from build123d import *

# Parameters (mm, degrees)
BOSS_EXTRUDE1_DEPTH = 5
SKETCH2_R           = 1.75
BOSS_EXTRUDE2_DEPTH = 6
CUT_EXTRUDE1_REACH  = 54.111
SKETCH3_R           = 1.75


with BuildPart() as part:
    # Sketch1 → Boss-Extrude1 (new body)
    with BuildSketch(Plane(origin=(0, 0, 0), x_dir=(1, 0, 0), z_dir=(0, 1, 0))):
        with BuildLine():
            Line((0, 0), (50, 0))
            Line((50, 0), (50, 11.2))
            Line((50, 11.2), (49.7, 11.2))
            ThreePointArc((49.7, 11.2), (49.38158785, 11.33158785), (49.25, 11.65))
            ThreePointArc((49.25, 11.65), (49.089793883, 12.579390672), (48.625, 13.4))
            Line((48.625, 13.4), (47.875, 13.4))
            ThreePointArc((47.875, 13.4), (47.410206117, 12.579390672), (47.25, 11.65))
            ThreePointArc((47.25, 11.65), (47.11841215, 11.33158785), (46.8, 11.2))
            Line((46.8, 11.2), (45.8, 11.2))
            ThreePointArc((45.8, 11.2), (45.48158785, 11.33158785), (45.35, 11.65))
            ThreePointArc((45.35, 11.65), (45.189793883, 12.579390672), (44.725, 13.4))
            Line((44.725, 13.4), (43.975, 13.4))
            ThreePointArc((43.975, 13.4), (43.510206117, 12.579390672), (43.35, 11.65))
            ThreePointArc((43.35, 11.65), (43.21841215, 11.33158785), (42.9, 11.2))
            Line((42.9, 11.2), (41.9, 11.2))
            ThreePointArc((41.9, 11.2), (41.58158785, 11.33158785), (41.45, 11.65))
            ThreePointArc((41.45, 11.65), (41.289793883, 12.579390672), (40.825, 13.4))
            Line((40.825, 13.4), (40.075, 13.4))
            ThreePointArc((40.075, 13.4), (39.610206117, 12.579390672), (39.45, 11.65))
            ThreePointArc((39.45, 11.65), (39.31841215, 11.33158785), (39, 11.2))
            Line((39, 11.2), (38, 11.2))
            ThreePointArc((38, 11.2), (37.68158785, 11.33158785), (37.55, 11.65))
            ThreePointArc((37.55, 11.65), (37.389793883, 12.579390672), (36.925, 13.4))
            Line((36.925, 13.4), (36.175, 13.4))
            ThreePointArc((36.175, 13.4), (35.710206117, 12.579390672), (35.55, 11.65))
            ThreePointArc((35.55, 11.65), (35.41841215, 11.33158785), (35.1, 11.2))
            Line((35.1, 11.2), (34.1, 11.2))
            ThreePointArc((34.1, 11.2), (33.78158785, 11.33158785), (33.65, 11.65))
            ThreePointArc((33.65, 11.65), (33.489793883, 12.579390672), (33.025, 13.4))
            Line((33.025, 13.4), (32.275, 13.4))
            ThreePointArc((32.275, 13.4), (31.810206117, 12.579390672), (31.65, 11.65))
            ThreePointArc((31.65, 11.65), (31.51841215, 11.33158785), (31.2, 11.2))
            Line((31.2, 11.2), (30.2, 11.2))
            ThreePointArc((30.2, 11.2), (29.88158785, 11.33158785), (29.75, 11.65))
            ThreePointArc((29.75, 11.65), (29.589793883, 12.579390672), (29.125, 13.4))
            Line((29.125, 13.4), (28.375, 13.4))
            ThreePointArc((28.375, 13.4), (27.910206117, 12.579390672), (27.75, 11.65))
            ThreePointArc((27.75, 11.65), (27.61841215, 11.33158785), (27.3, 11.2))
            Line((27.3, 11.2), (26.3, 11.2))
            ThreePointArc((26.3, 11.2), (25.98158785, 11.33158785), (25.85, 11.65))
            ThreePointArc((25.85, 11.65), (25.689793883, 12.579390672), (25.225, 13.4))
            Line((25.225, 13.4), (24.475, 13.4))
            ThreePointArc((24.475, 13.4), (24.010206117, 12.579390672), (23.85, 11.65))
            ThreePointArc((23.85, 11.65), (23.71841215, 11.33158785), (23.4, 11.2))
            Line((23.4, 11.2), (22.4, 11.2))
            ThreePointArc((22.4, 11.2), (22.08158785, 11.33158785), (21.95, 11.65))
            ThreePointArc((21.95, 11.65), (21.789793883, 12.579390672), (21.325, 13.4))
            Line((21.325, 13.4), (20.575, 13.4))
            ThreePointArc((20.575, 13.4), (20.110206117, 12.579390672), (19.95, 11.65))
            ThreePointArc((19.95, 11.65), (19.81841215, 11.33158785), (19.5, 11.2))
            Line((19.5, 11.2), (18.5, 11.2))
            ThreePointArc((18.5, 11.2), (18.18158785, 11.33158785), (18.05, 11.65))
            ThreePointArc((18.05, 11.65), (17.889793883, 12.579390672), (17.425, 13.4))
            Line((17.425, 13.4), (16.675, 13.4))
            ThreePointArc((16.675, 13.4), (16.210206117, 12.579390672), (16.05, 11.65))
            ThreePointArc((16.05, 11.65), (15.91841215, 11.33158785), (15.6, 11.2))
            Line((15.6, 11.2), (14.6, 11.2))
            ThreePointArc((14.6, 11.2), (14.28158785, 11.33158785), (14.15, 11.65))
            ThreePointArc((14.15, 11.65), (13.989793883, 12.579390672), (13.525, 13.4))
            Line((13.525, 13.4), (12.775, 13.4))
            ThreePointArc((12.775, 13.4), (12.310206117, 12.579390672), (12.15, 11.65))
            ThreePointArc((12.15, 11.65), (12.01841215, 11.33158785), (11.7, 11.2))
            Line((11.7, 11.2), (10.7, 11.2))
            ThreePointArc((10.7, 11.2), (10.38158785, 11.33158785), (10.25, 11.65))
            ThreePointArc((10.25, 11.65), (10.089793883, 12.579390672), (9.625, 13.4))
            Line((9.625, 13.4), (8.875, 13.4))
            ThreePointArc((8.875, 13.4), (8.410206117, 12.579390672), (8.25, 11.65))
            ThreePointArc((8.25, 11.65), (8.11841215, 11.33158785), (7.8, 11.2))
            Line((7.8, 11.2), (6.8, 11.2))
            ThreePointArc((6.8, 11.2), (6.48158785, 11.33158785), (6.35, 11.65))
            ThreePointArc((6.35, 11.65), (6.189793883, 12.579390672), (5.725, 13.4))
            Line((5.725, 13.4), (4.975, 13.4))
            ThreePointArc((4.975, 13.4), (4.510206117, 12.579390672), (4.35, 11.65))
            ThreePointArc((4.35, 11.65), (4.21841215, 11.33158785), (3.9, 11.2))
            Line((3.9, 11.2), (2.9, 11.2))
            ThreePointArc((2.9, 11.2), (2.58158785, 11.33158785), (2.45, 11.65))
            ThreePointArc((2.45, 11.65), (2.289793883, 12.579390672), (1.825, 13.4))
            Line((1.825, 13.4), (1.075, 13.4))
            ThreePointArc((1.075, 13.4), (0.610206117, 12.579390672), (0.45, 11.65))
            ThreePointArc((0.45, 11.65), (0.31841215, 11.33158785), (0, 11.2))
            Line((0, 11.2), (0, 0))
        make_face()
    extrude(amount=BOSS_EXTRUDE1_DEPTH)

    # Sketch2 → Boss-Extrude2 (add)
    # profile 1 of 2: a face of its own
    with BuildSketch(Plane.XZ):
        with BuildLine():
            Line((12, -7.5), (8, -7.5))
            ThreePointArc((8, -7.5), (5.5, -5), (8, -2.5))
            Line((8, -2.5), (12, -2.5))
            ThreePointArc((12, -2.5), (14.5, -5), (12, -7.5))
        make_face()
        with Locations(Location((10, -5, 0), (0, 0, 270))):
            Circle(SKETCH2_R, mode=Mode.SUBTRACT)
    # profile 2 of 2: a face of its own
    with BuildSketch(Plane.XZ):
        with BuildLine():
            Line((42, -7.5), (38, -7.5))
            ThreePointArc((38, -7.5), (35.5, -5), (38, -2.5))
            Line((38, -2.5), (42, -2.5))
            ThreePointArc((42, -2.5), (44.5, -5), (42, -7.5))
        make_face()
        with Locations(Location((40, -5, 0), (0, 0, 270))):
            Circle(SKETCH2_R, mode=Mode.SUBTRACT)
    extrude(amount=BOSS_EXTRUDE2_DEPTH)

    # Sketch3 → Cut-Extrude1 (cut, up to next)
    with BuildSketch(Plane.XZ, mode=Mode.PRIVATE) as cut_extrude1_sk1:
        with Locations(Location((40, -5, 0), (0, 0, 270))):
            Circle(SKETCH3_R)
    cut_extrude1_tool1 = extrude(cut_extrude1_sk1.sketch, amount=-CUT_EXTRUDE1_REACH, mode=Mode.PRIVATE) & part.part
    # Sketch3 → Cut-Extrude1 (cut, up to next)
    with BuildSketch(Plane.XZ, mode=Mode.PRIVATE) as cut_extrude1_sk2:
        with Locations(Location((10, -5, 0), (0, 0, 270))):
            Circle(SKETCH3_R)
    cut_extrude1_tool2 = extrude(cut_extrude1_sk2.sketch, amount=-CUT_EXTRUDE1_REACH, mode=Mode.PRIVATE) & part.part
    add(cut_extrude1_tool1.solids().sort_by_distance((40, 0, -5))[0], mode=Mode.SUBTRACT)
    add(cut_extrude1_tool2.solids().sort_by_distance((10, 0, -5))[0], mode=Mode.SUBTRACT)


solid = part.part
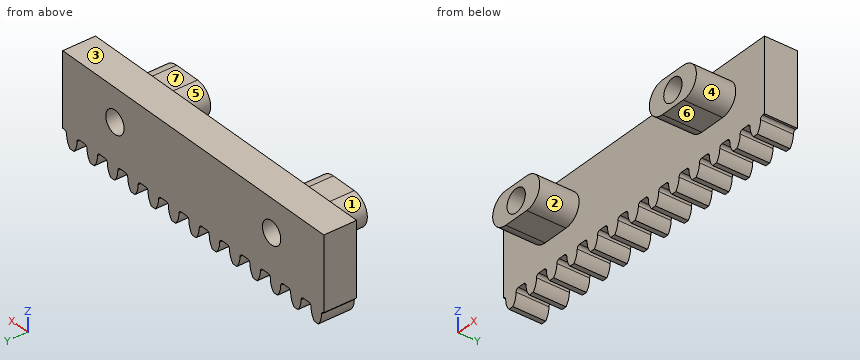
Build history of the part. All positions in model axes, mm. Face numbers are marked on the shaded views. A direction names the side the tool comes from. Round coordinates to 2 decimals unless told otherwise and drop trailing zeros. Loops run counter-clockwise (first coordinate to the right, second up) from the corner with the lowest first, then second, coordinate; pieces in that order, holes last. Notation, with made-up numbers: (-33, 27) -> (1, 27) arc R12 cw to (1, 39) -> close; hole circle Ø4 at (77, -19). An arc over 180 degrees is marked (long way). Answer in a Markdown table with one row per item.
Item 1: Mould opens along X. For the marked faces 1, 2 and 3 say: +X half, -X half, draft (parallel to the pull), parting line (faces both ways), or undercut.
Answers below:
| item | result |
|---|---|
| face 1 | -X half |
| face 2 | undercut |
| face 3 | draft |
Item 2: Saw through at C-C (y = 3). State how many separate pieces and enclosed holes the cut face has, and give its area (3 significant figures).
Answers below:
| item | result |
|---|---|
| separate pieces | 1 |
| enclosed holes | 2 |
| area | 590 mm² |
Item 3: Saw through at A-A (z = -5). Write the cut outline in (x, y), and give its area (3 significant figures).
Answers below:
| item | result |
|---|---|
| outline | (0, 0) -> (5.5, 0) -> (5.5, -6) -> (8.25, -6) -> (8.25, 5) -> (0, 5) -> close; (11.75, -6) -> (14.5, -6) -> (14.5, 0) -> (35.5, 0) -> (35.5, -6) -> (38.25, -6) -> (38.25, 5) -> (11.75, 5) -> close; (41.75, -6) -> (44.5, -6) -> (44.5, 0) -> (50, 0) -> (50, 5) -> (41.75, 5) -> close |
| area | 281 mm² |
Item 4: Saw through at B-B (y = -4.5). Write the cut outline in (x, z), and give its area (3 significant figures).
Answers below:
| item | result |
|---|---|
| outline | (8, -7.5) -> (12, -7.5) arc R2.5 ccw to (12, -2.5) -> (8, -2.5) arc R2.5 ccw to start; (38, -7.5) -> (42, -7.5) arc R2.5 ccw to (42, -2.5) -> (38, -2.5) arc R2.5 ccw to start; hole circle Ø3.5 at (10, -5); hole circle Ø3.5 at (40, -5) |
| area | 60.0 mm² |
Item 5: Drill centre lines: L1, parallel to X at y = 2.55, z = -5; L2, parallel to X at y = -4.75, z = -5; L3, parallel to Y at x = 15.5, z = -7. Where is each one in solid material? Low to high. Write a range as [from, to].
Answers below:
| item | result |
|---|---|
| L1 | x = [0, 8.25], [11.75, 38.25], [41.75, 50] |
| L2 | x = [5.5, 8.25], [11.75, 14.5], [35.5, 38.25], [41.75, 44.5] |
| L3 | y = [0, 5] |
Item 6: Pin check, flat tips, straight feed: pin 1 (0.5 mm diameter, centred on x = 7.5, y = 1.5, fed in from -Z); pin 2 (3 mm diameter, centred on x = 19.5, z = -4, fed in from -Y); pin 3 (1.2 mm diameter, centred on x = 40, y = -2, fed in from -Z). Stop position of each tip, or through.
Answers below:
| item | result |
|---|---|
| pin 1 | stops at z = -11.2 |
| pin 2 | stops at y = 0 |
| pin 3 | stops at z = -7.5 |
Item 7: Which spindle directions (+Z, -Z, +X, -X, +Y, -Y) get a long thin tool onto all of the face, cutting with end or side? Do the marked faces 4, 5, 6 and 7. Say none if no direction does.
Answers below:
| item | result |
|---|---|
| face 4 | +X, -Y |
| face 5 | -Y |
| face 6 | -Z, +X, -X, -Y |
| face 7 | +Z, +X, -X, -Y |
Item 8: Saw through at D-D (z = -9.25). Write the cut outline in (x, y).
Answers below:
| item | result |
|---|---|
| outline | (0, 0) -> (50, 0) -> (50, 5) -> (0, 5) -> close |
